from build123d import *

# Parameters (mm, degrees)
SKETCH_2_W               = 180
SKETCH_2_H               = 90
SM_BASE_FLANGE_1_DEPTH   = 2
SM_START                 = -90
SM_EDGE_FLANGE_1_DEPTH   = 180
SM_EDGE_FLANGE_1_2_DEPTH = 180
SKETCH_10_W              = 100
SKETCH_10_H              = 42.023300627
CUT_EXTRUDE_1_DEPTH      = 10
SKETCH_11_R              = 2.1
CUT_EXTRUDE_2_DEPTH      = 2
SKETCH_12_W              = 25
SKETCH_12_H              = 26.58587188
CUT_EXTRUDE_3_DEPTH      = 10
SKETCH_13_R              = 2.1
SKETCH_13_R_2            = 2.090991101
CUT_EXTRUDE_4_DEPTH      = 10
SKETCH_14_R              = 4
CUT_EXTRUDE_5_DEPTH      = 1


# Read off the part's stored shape, not the designer's step: 边线-法兰1
# Sheet-metal steps are written as plain solids
with BuildPart() as part:
    # Sketch 2 → 基体-法兰1 (new body)
    with BuildSketch(Plane.XY):
        Rectangle(SKETCH_2_W, SKETCH_2_H)
    extrude(amount=-SM_BASE_FLANGE_1_DEPTH)

    # 边线-法兰1 outline → 边线-法兰1 (cut)
    with BuildSketch(Plane.YZ.offset(SM_START)):
        with BuildLine():
            Line((-45, -2), (-44.922280112, -2))
            ThreePointArc((-44.922280112, -2), (-42.669051938, -0.519259301), (-40.023300627, 0))
            Line((-40.023300627, 0), (-45, 0))
            Line((-45, 0), (-45, -2))
        make_face()
    extrude(amount=SM_EDGE_FLANGE_1_DEPTH, mode=Mode.SUBTRACT)

    # Sm Edge Flange 1 2 outline → Sm Edge Flange 1 2 (add)
    with BuildSketch(Plane.YZ.offset(SM_START)):
        with BuildLine():
            ThreePointArc((-44.922280112, -2), (-45.242255885, -2.334969881), (-45.539375902, -2.690369673))
            Line((-45.539375902, -2.690369673), (-61.907273007, -23.640322608))
            Line((-61.907273007, -23.640322608), (-60.3312515, -24.871645559))
            Line((-60.3312515, -24.871645559), (-43.963354395, -3.921692623))
            ThreePointArc((-43.963354395, -3.921692623), (-42.215156361, -2.506029769), (-40.023300627, -2))
            Line((-40.023300627, -2), (-44.922280112, -2))
        make_face()
    extrude(amount=SM_EDGE_FLANGE_1_2_DEPTH)

    # 草图10 → 切除-拉伸1 (cut)
    with BuildSketch(Plane(origin=(0, 0, -2), x_dir=(-1, 0, 0), z_dir=(0, 0, -1))):
        with Locations((0, -6.011650313)):
            Rectangle(SKETCH_10_W, SKETCH_10_H)
    extrude(amount=-CUT_EXTRUDE_1_DEPTH, mode=Mode.SUBTRACT)

    # 草图11 → 切除-拉伸2 (cut)
    with BuildSketch(Plane(origin=(0, -26.972946925, 21.073575737), x_dir=(1, 0, 0), z_dir=(0, -0.788010753606719, 0.6156614753256621))):
        with Locations(Location((60, -43.742751467, 0), (0, 0, 270))):
            Circle(SKETCH_11_R)
        with Locations(Location((20, -43.742751467, 0), (0, 0, 270))):
            Circle(SKETCH_11_R)
        with Locations(Location((-20, -43.742751467, 0), (0, 0, 90))):
            Circle(SKETCH_11_R)
        with Locations(Location((-60, -43.742751467, 0), (0, 0, 90))):
            Circle(SKETCH_11_R)
    extrude(amount=-CUT_EXTRUDE_2_DEPTH, mode=Mode.SUBTRACT)

    # 草图12 → 切除-拉伸3 (cut)
    with BuildSketch(Plane(origin=(0, -25.396925418, 19.842252786), x_dir=(1, 0, 0), z_dir=(0, 0.788010753606719, -0.6156614753256621))):
        with Locations((-77.5, 43.449815527)):
            Rectangle(SKETCH_12_W, SKETCH_12_H)
        with Locations((77.5, 43.449815527)):
            Rectangle(SKETCH_12_W, SKETCH_12_H)
    extrude(amount=-CUT_EXTRUDE_3_DEPTH, mode=Mode.SUBTRACT)

    # 草图13 → 切除-拉伸4 (cut)
    with BuildSketch(Plane(origin=(0, 0, -2), x_dir=(-1, 0, 0), z_dir=(0, 0, -1))):
        with Locations((50, 30)):
            Circle(SKETCH_13_R)
        with Locations((50, 40)):
            Circle(SKETCH_13_R)
        with Locations((-50, 30)):
            Circle(SKETCH_13_R)
        with Locations((-50, 40)):
            Circle(SKETCH_13_R_2)
    extrude(amount=-CUT_EXTRUDE_4_DEPTH, mode=Mode.SUBTRACT)

    # 草图14 → 切除-拉伸5 (cut)
    with BuildSketch(Plane.XY):
        with Locations((-50, 40)):
            Circle(SKETCH_14_R)
        with Locations((-50, 30)):
            Circle(SKETCH_14_R)
        with Locations((50, 40)):
            Circle(SKETCH_14_R)
        with Locations((50, 30)):
            Circle(SKETCH_14_R)
    extrude(amount=-CUT_EXTRUDE_5_DEPTH, mode=Mode.SUBTRACT)


solid = part.part
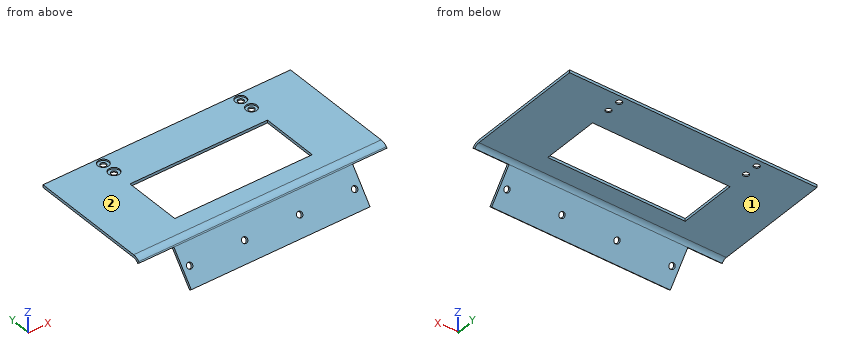
Check sheet for the modelled part. Datum: model origin and axes. Units: mm. Face numbers are marked on the shaded views. A direction names the side the tool comes from. Coordinates: 2 decimals unless noted, no trailing zeros. Loops run counter-clockwise (first coordinate to the right, second up) from the corner with the lowest first, then second, coordinate; pieces in that order, holes last. Notation, with made-up numbers: (-16.75, -21) -> (14.25, -21) arc R28 cw to (14.25, 14) -> close; hole circle Ø1 at (68.5, 18). An arc over 180 degrees is marked (long way). Write item = value, one per line. Start each with the question number.
1. Material ranges on line 1 (X direction, y = -13, z = -1.25); line 2 (Z direction, x = 1, y = 39); line 3 (X direction, y = -52, z = -11.25), recorded low to high.
2. Depth check by flat-ended pin: P1, Ø2.5, axis at x = 51.5, y = 41, coming from the +Z side; P2, Ø14.5, axis at y = -57, z = -18, coming from the +X side; P3, Ø2, axis at x = -60, z = -9, coming from the +Y side. Enter the tip coordinate at first touch or a pass-through.
3. Section check D-D on z = -8. Record the cut outline in (x, y).
4. Section check A-A on y = 40. Record the cut outline in (x, z).
5. Tool access check on the marked faces 1 and 2. Record the directions out of +Z, -Z, +X, -X, +Y, -Y that give a thin tool (end or side, any length) a straight path to the whole face; none if there is none.
6. Section check B-B on y = -21.5. Record the cut outline in (x, z).
7. Section check C-C on x = 28. Record the cut outline in (y, z), then the cut area to 3 significant figures.
Responses:
q1.line_1 = -90 to -50, 50 to 90
q1.line_2 = -2 to 0
q1.line_3 = -65 to 65
q2.P1 = -1
q2.P2 = 65
q2.P3 = -47.15
q3.outline = (-65, -49.69) -> (65, -49.69) -> (65, -47.15) -> (-65, -47.15) -> close
q4.outline = (-90, -2) -> (-52.1, -2) -> (-52.1, -1) -> (-54, -1) -> (-54, 0) -> (-90, 0) -> close; (-47.9, -2) -> (47.91, -2) -> (47.91, -1) -> (46, -1) -> (46, 0) -> (-46, 0) -> (-46, -1) -> (-47.9, -1) -> close; (52.09, -2) -> (90, -2) -> (90, 0) -> (54, 0) -> (54, -1) -> (52.09, -1) -> close
q5.face_1 = -Z, +X, -X, +Y
q5.face_2 = +Z, +X, -X, +Y, -Y
q6.outline = (-90, -2) -> (-50, -2) -> (-50, 0) -> (-90, 0) -> close; (50, -2) -> (90, -2) -> (90, 0) -> (50, 0) -> close
q7.outline = (-61.91, -23.64) -> (-60.33, -24.87) -> (-43.96, -3.92) arc R5 cw to (-40.02, -2) -> (-27.02, -2) -> (-27.02, 0) -> (-40.02, 0) arc R7 ccw to (-45.54, -2.69) -> close; (15, -2) -> (45, -2) -> (45, 0) -> (15, 0) -> close
q7.area = 150 mm2
